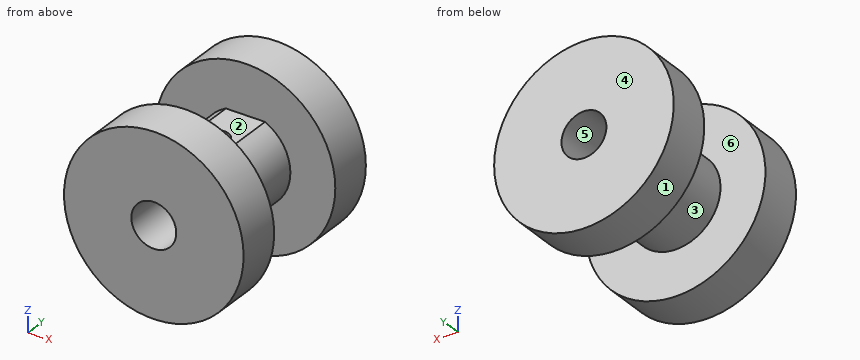
from build123d import *

# Parameters (mm, degrees)
SKETCH1_R           = 10
SKETCH1_R_2         = 5
SKETCH1_R_3         = 2.5
BOSS_EXTRUDE1_DEPTH = 10
SKETCH1_3_R         = 10
SKETCH1_3_R_2       = 5
CUT_EXTRUDE1_DEPTH  = 5
CUT_EXTRUDE2_REACH  = 16.5
SKETCH4_R           = 1.5


with BuildPart() as part:
    # Sketch1 → Boss-Extrude1 (new body, symmetric)
    with BuildSketch(Plane(origin=(0, 0, 0), x_dir=(1, 0, 0), z_dir=(0, 1, 0))):
        Circle(SKETCH1_R)
        Circle(SKETCH1_R_2, mode=Mode.SUBTRACT)
        Circle(SKETCH1_R_2)
        Circle(SKETCH1_R_3, mode=Mode.SUBTRACT)
        with BuildLine():
            Line((2.179449472, -4.5), (-2.179449472, -4.5))
            ThreePointArc((-2.179449472, -4.5), (0, -5), (2.179449472, -4.5))
        make_face()
    extrude(amount=BOSS_EXTRUDE1_DEPTH, both=True)

    # Sketch1_3 → Cut-Extrude1 (cut, symmetric)
    with BuildSketch(Plane(origin=(0, 0, 0), x_dir=(1, 0, 0), z_dir=(0, 1, 0))):
        Circle(SKETCH1_3_R)
        Circle(SKETCH1_3_R_2, mode=Mode.SUBTRACT)
        with BuildLine():
            Line((2.179449472, -4.5), (-2.179449472, -4.5))
            ThreePointArc((-2.179449472, -4.5), (0, -5), (2.179449472, -4.5))
        make_face()
    extrude(amount=CUT_EXTRUDE1_DEPTH, both=True, mode=Mode.SUBTRACT)

    # Sketch4 → Cut-Extrude2 (cut, up to next)
    with BuildSketch(Plane.XY.offset(4.5), mode=Mode.PRIVATE) as cut_extrude2_sk1:
        Circle(SKETCH4_R)
    cut_extrude2_tool1 = extrude(cut_extrude2_sk1.sketch, amount=-CUT_EXTRUDE2_REACH, mode=Mode.PRIVATE) & part.part
    add(cut_extrude2_tool1.solids().sort_by_distance((0, 0, 4.5))[0], mode=Mode.SUBTRACT)


solid = part.part
Geometry: final body of the model. Coordinates: model frame, mm. Face numbers are marked on the shaded views. A direction names the side the tool comes from. Coordinates: 2 decimals unless noted, no trailing zeros. Write each loop counter-clockwise with the first axis right and the second up, starting at its lowest first coordinate (ties: lowest second). Pieces come first, ordered by that corner, then holes. Notation, with made-up numbers: (-27, -22.5) - (-11, -22.5) arc R13 ccw to (-11, -9.5) - close; hole circle Ø1 at (35, 8). An arc over 180 degrees is marked (long way). Return JSON: item names as keys, results as strings.
Item 1: Pin query (flat end, axial travel): pin 1 Ø5 at (x, y) = (0, 0) entering from +Z; pin 2 Ø4.5 at (x, z) = (0, 0) entering from -Y; pin 3 Ø8 at (x, y) = (-6.5, -3.5) entering from +Z; pin 4 Ø1 at (x, y) = (4, 7) entering from -Z. Return the tip coordinate at first contact, or that it passes through.
Completed:
{"pin 1": "stops at z = 4.5", "pin 2": "passes through", "pin 3": "stops at z = 9.6", "pin 4": "stops at z = -9.37"}
Item 2: Section query A-A (x = 0). Output: boundary loops of the cut face in (y, z).
Completed:
{"outline": "(-10, -10) - (-5, -10) - (-5, -5) - (5, -5) - (5, -10) - (10, -10) - (10, -2.5) - (-10, -2.5) - close; (-10, 2.5) - (-1.5, 2.5) - (-1.5, 4.5) - (-5, 4.5) - (-5, 10) - (-10, 10) - close; (1.5, 2.5) - (10, 2.5) - (10, 10) - (5, 10) - (5, 4.5) - (1.5, 4.5) - close"}
Item 3: Pull-direction query (Y, two-part tool) for the marked faces 4, 5 and 6; classes: +Y half, -Y half, draft (parallel to the pull), parting line (faces both ways), or undercut.
Completed:
{"face 4": "+Y half", "face 5": "draft", "face 6": "undercut"}
Item 4: Line query: L1, parallel to Y at x = 4, z = -5.5; L2, parallel to X at y = 4.25, z = 0; L3, parallel to X at y = 0, z = 3.55. Output: solid intervals per line, ascending.
Completed:
{"L1": "y = -10 to -5, 5 to 10", "L2": "x = -5 to -2.5, 2.5 to 5", "L3": "x = -3.52 to -1.5, 1.5 to 3.52"}
Item 5: Reachability of the marked faces 1, 2 and 3 from +Z, -Z, +X, -X, +Y, -Y: full face, straight path, thin tool, end or side. Return the list, or none.
Completed:
{"face 1": "+Y, -Y", "face 2": "+Z, +X, -X", "face 3": "none"}
Item 6: Section query D-D (y = 0). Output: boundary loops of the cut face in (x, z), and give its area (3 significant figures).
Completed:
{"outline": "(-2.18, 4.5) arc R5 ccw (long way) to (2.18, 4.5) - (1.5, 4.5) - (1.5, 2) arc R2.5 cw (long way) to (-1.5, 2) - (-1.5, 4.5) - close", "area": "51.0 mm2"}
Item 7: Section query C-C (x = 7). Output: boundary loops of the cut face in (y, z), and give its area (3 significant figures).
Completed:
{"outline": "(-10, -7.14) - (-5, -7.14) - (-5, 7.14) - (-10, 7.14) - close; (5, -7.14) - (10, -7.14) - (10, 7.14) - (5, 7.14) - close", "area": "143 mm2"}
Item 8: Section query B-B (z = 0). Output: boundary loops of the cut face in (x, y), and give its area (3 significant figures).
Completed:
{"outline": "(-10, -10) - (-2.5, -10) - (-2.5, 10) - (-10, 10) - (-10, 5) - (-5, 5) - (-5, -5) - (-10, -5) - close; (2.5, -10) - (10, -10) - (10, -5) - (5, -5) - (5, 5) - (10, 5) - (10, 10) - (2.5, 10) - close", "area": "200 mm2"}
